```python
from build123d import *

# Parameters (mm, degrees)
SKETCH1_R                      = 76.2
BOSS_EXTRUDE1_DEPTH            = 3.175
SKETCH2_R                      = 12.065
BOSS_EXTRUDE2_DEPTH            = 3.175
SKETCH5_R                      = 10.4
CUT_EXTRUDE1_DEPTH             = 5.525
SKETCH6_R                      = 5
CUT_EXTRUDE2_DEPTH             = 4
CBORE_FOR_M2_SHCS1_D           = 2.2
CBORE_FOR_M2_SHCS1_DEPTH       = 6
CBORE_FOR_M2_SHCS1_CBORE_D     = 4.4
CBORE_FOR_M2_SHCS1_CBORE_DEPTH = 2
CBORE_FOR_M2_SHCS1_TIP         = 0.660946681
M4_CLEARANCE_HOLE1_D           = 4.5
M5_CLEARANCE_HOLE1_D           = 5.5


with BuildPart() as part:
    # Sketch1 → Boss-Extrude1 (new, symmetric)
    with BuildSketch(Plane(origin=(0, 0, 0), x_dir=(1, 0, 0), z_dir=(0, 1, 0))):
        with Locations(Location((0, 0, 0), (0, 0, 270))):
            Circle(SKETCH1_R)
    extrude(amount=BOSS_EXTRUDE1_DEPTH, both=True)

    # Sketch2 → Boss-Extrude2 (add)
    with BuildSketch(Plane.XZ.offset(3.175)):
        with Locations(Location((0, 0, 0), (0, 0, 270))):
            Circle(SKETCH2_R)
    extrude(amount=BOSS_EXTRUDE2_DEPTH)

    # Sketch5 → Cut-Extrude1 (cut)
    with BuildSketch(Plane(origin=(0, 3.175, 0), x_dir=(1, 0, 0), z_dir=(0, 1, 0))):
        with Locations(Location((0, 0, 0), (0, 0, 270))):
            Circle(SKETCH5_R)
    extrude(amount=-CUT_EXTRUDE1_DEPTH, mode=Mode.SUBTRACT)

    # Sketch6 → Cut-Extrude2 (cut)
    with BuildSketch(Plane(origin=(0, -2.35, 0), x_dir=(1, 0, 0), z_dir=(0, 1, 0))):
        with Locations(Location((0, 0, 0), (0, 0, 270))):
            Circle(SKETCH6_R)
    extrude(amount=-CUT_EXTRUDE2_DEPTH, mode=Mode.SUBTRACT)

    # CBORE for M2 SHCS1
    with Locations(Plane(origin=(0, -2.35, 0), x_dir=(1, 0, 0), z_dir=(0, 1, 0))):
        with Locations((-5.65685425, 5.65685425), (0, 8), (5.65685425, 5.65685425), (8, 0), (5.65685425, -5.65685425), (0, -8), (-5.65685425, -5.65685425), (-8, 0)):
            CounterBoreHole(CBORE_FOR_M2_SHCS1_D / 2, CBORE_FOR_M2_SHCS1_CBORE_D / 2, CBORE_FOR_M2_SHCS1_CBORE_DEPTH, depth=CBORE_FOR_M2_SHCS1_DEPTH)
            with Locations((0, 0, -(CBORE_FOR_M2_SHCS1_DEPTH + CBORE_FOR_M2_SHCS1_TIP / 2))):  # 118° drill point
                Cone(0, CBORE_FOR_M2_SHCS1_D / 2, CBORE_FOR_M2_SHCS1_TIP, mode=Mode.SUBTRACT)

    # M4 Clearance Hole1 (through all)
    with Locations(Plane(origin=(0, 3.175, 0), x_dir=(1, 0, 0), z_dir=(0, 1, 0))):
        with Locations((19.05, -44.388212048), (-19.05, -44.388212048)):
            Hole(M4_CLEARANCE_HOLE1_D / 2)

    # M5 Clearance Hole1 (through all)
    with Locations(Plane(origin=(0, 3.175, 0), x_dir=(1, 0, 0), z_dir=(0, 1, 0))):
        with Locations((-33.6688086, 31.567387952), (-14.6188086, 31.567387952), (4.4311914, 31.567387952), (-15.875, -19.249706448), (15.875, -19.249706448)):
            Hole(M5_CLEARANCE_HOLE1_D / 2)


solid = part.part
```
Geometry check sheet. Reference: the model listing, model coordinates, mm. A direction names the side the tool comes from. Coordinates: 2 decimals unless noted, no trailing zeros. Loops run counter-clockwise (first coordinate to the right, second up) from the corner with the lowest first, then second, coordinate; pieces in that order, holes last.
Item 1: Access from +Z, -Z, +X, -X, +Y, -Y to the whole of each face (thin tool, end or side, straight path). Record for faces 3 (the face through (3.12, 0.45, 9.92)), 4 (the face through (1, 3.175, 16)).
Item 2: Sectioned sample at A-A, the plane x = 31.5. Record the boundary of the cut face in (y, z) (3 decimals), then the cut area to 3 significant figures.
Item 3: Sectioned sample at B-B, the plane z = 29.5. Record the boundary of the cut face in (x, y) (3 decimals), then the cut area to 3 significant figures.
Item 4: Thickness scan on line 1 (X direction, y = -5.5, z = -6); line 2 (Y direction, x = -40, z = 36.5) (3 decimals); line 3 (X direction, y = 1.5, z = -30.5). Record the ranges inside material, lowest first.
Item 5: Release check for a two-part mould opening along X. For faces 1 (the face through (1, -3.175, 16)), 2 (the face through (-7, -4.35, 6)) record: released by +X, released by -X, zero draft, split by the parting line, or undercut.
Item 6: Go/stop test with flat-tipped pins: pin 1 Ø1.3 at (x, z) = (5.5, 6) entering from +Y; pin 2 Ø2 at (x, y) = (-38, -2.5) entering from -Z; pin 3 Ø4 at (x, z) = (0, 8) entering from +Y; pin 4 Ø1 at (x, z) = (-2.5, -59.5) entering from -Y (3 decimals). Record where each tip stops, or that it passes through.
Check result:
1. face 3: +Y
1. face 4: +Z, -Z, +X, -X, +Y
2. outline: (-3.175, -69.384) - (3.175, -69.384) - (3.175, 69.384) - (-3.175, 69.384) - close
2. area: 881 mm2
3. outline: (-70.258, -3.175) - (70.258, -3.175) - (70.258, 3.175) - (-70.258, 3.175) - close
3. area: 892 mm2
4. line 1: x = -10.47 to -6.7, -4.61 to 4.61, 6.7 to 10.47
4. line 2: y = -3.175 to 3.175
4. line 3: x = -69.83 to -36.2, -31.13 to -17.15, -12.08 to 1.9, 6.97 to 69.83
5. face 1: zero draft
5. face 2: undercut
6. pin 1: passes through
6. pin 2: stops at z = -66.61
6. pin 3: stops at y = -4.35
6. pin 4: stops at y = -3.175
